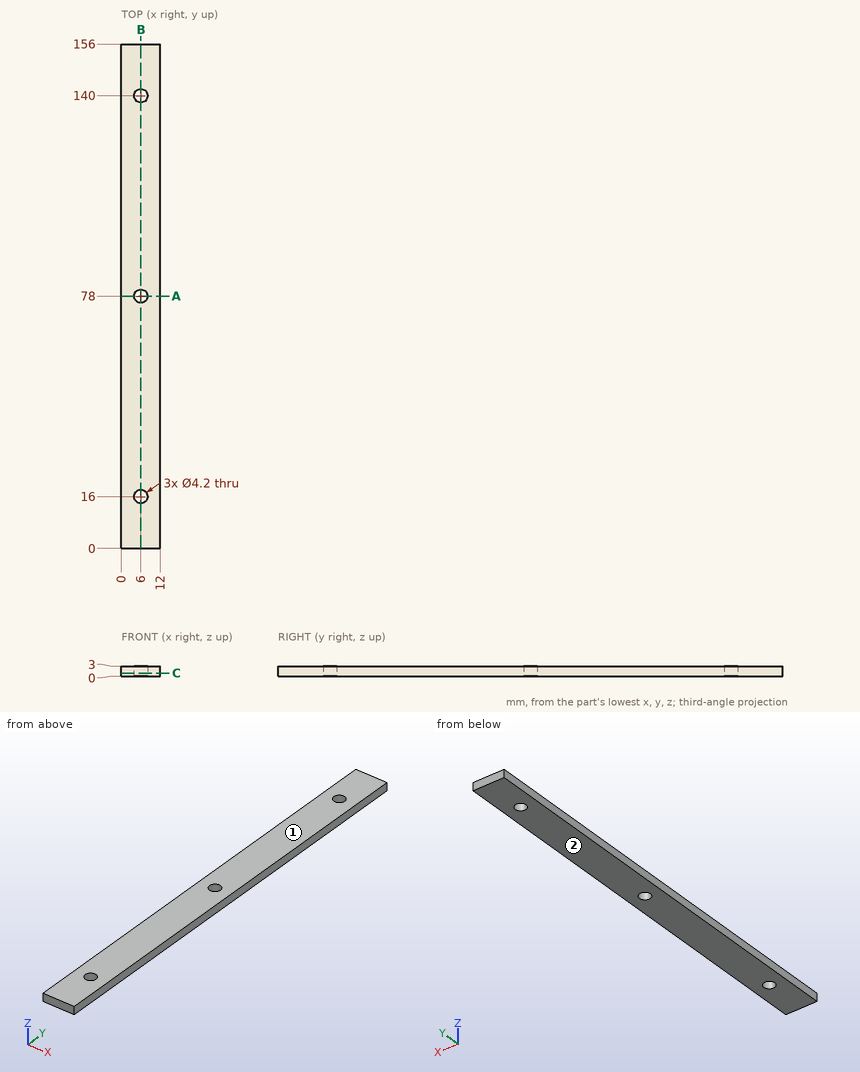
Source: three-view drawing plus pictorial views. Frame: mm from the lowest corner of the part. Round coordinates to 2 decimals unless told otherwise and drop trailing zeros. Loops run counter-clockwise (first coordinate to the right, second up) from the corner with the lowest first, then second, coordinate; pieces in that order, holes last.
Q1. Section B-B on x = 6. Return loops of the section in (y, z).
Q2. Section C-C on z = 0.9. Return loops of the section in (x, y).
Q3. Section A-A on y = 78. Return loops of the section in (x, z).
Q4. Material intervals for L1, parallel to Y at x = 6, z = 1.45; L2, parallel to Y at x = 4.5, z = 1.1; L3, parallel to X at y = 140, z = 1.25, sorted ascending.
Q5. Pull-direction query (Z, two-part tool) for the marked faces 1 and 2; classes: released by +Z, released by -Z, zero draft, split by the parting line, or undercut.
Evaluation:
1. outline: (0, 0) - (13.9, 0) - (13.9, 3) - (0, 3) - close; (18.1, 0) - (75.9, 0) - (75.9, 3) - (18.1, 3) - close; (80.1, 0) - (137.9, 0) - (137.9, 3) - (80.1, 3) - close; (142.1, 0) - (156, 0) - (156, 3) - (142.1, 3) - close
2. outline: (0, 0) - (12, 0) - (12, 156) - (0, 156) - close; hole circle Ø4.2 at (6, 16); hole circle Ø4.2 at (6, 78); hole circle Ø4.2 at (6, 140)
3. outline: (0, 0) - (3.9, 0) - (3.9, 3) - (0, 3) - close; (8.1, 0) - (12, 0) - (12, 3) - (8.1, 3) - close
4. L1: y = 0 to 13.9, 18.1 to 75.9, 80.1 to 137.9, 142.1 to 156
4. L2: y = 0 to 14.53, 17.47 to 76.53, 79.47 to 138.53, 141.47 to 156
4. L3: x = 0 to 3.9, 8.1 to 12
5. face 1: released by +Z
5. face 2: released by -Z
